Autodesk Inventor part; units mm, degrees
ref_plane "YZ Plane" through (0, 0, 0) normal (1, 0, 0) x (0, 1, 0)
ref_plane "XZ Plane" through (0, 0, 0) normal (0, 1, 0) x (-1, 0, 0)
ref_plane "XY Plane" through (0, 0, 0) normal (0, 0, 1) x (1, 0, 0)
sketch "Sketch1" plane through (0, 0, 0) normal (0, 1, 0) x (-1, 0, 0)
  circle A0 centre (0, 0) radius 25
  line L0 (10, 1.5) -> (-10, 1.5)
  line L1 (-10, 1.5) -> (-10, -1.5)
  line L2 (-10, -1.5) -> (10, -1.5)
  line L3 (10, -1.5) -> (10, 1.5)
  line L4 (1.5, 10) -> (-1.5, 10)
  line L5 (-1.5, 10) -> (-1.5, -10)
  line L6 (-1.5, -10) -> (1.5, -10)
  line L7 (1.5, -10) -> (1.5, 10)
  point P0 (-1.5, 1.5)
  point P1 (1.5, 1.5)
  point P2 (1.5, -1.5)
  point P3 (-1.5, -1.5)
  dimension "d0" = 50
  dimension "d1" = 20
  dimension "d2" = 3
  dimension "d3" = 1.5
  dimension "d4" = 10
  dimension "d5" = 3
  dimension "d6" = 20
  dimension "d7" = 10
  dimension "d8" = 1.5
extrude "Extrusion1" add sketch "Sketch1" along normal blind 3
properties part number "Base Arvore"
Verification items for the finished model (mm, model axes). A direction names the side the tool comes from. Give positions to 0.01 mm unless a question says otherwise; leave off trailing zeros. Write each loop counter-clockwise with the first axis right and the second up, starting at its lowest first coordinate (ties: lowest second). Pieces come first, ordered by that corner, then holes. Notation, with made-up numbers: (59.25, 7.25) - (82.25, 7.25) arc R10 ccw to (82.25, 22.25) - close; hole circle Ø9 at (10.5, 66.25). An arc over 180 degrees is marked (long way). Put each result on its own line as item: value.
Q1. Section check A-A on x = 0. Record the cut outline in (y, z).
Result:
outline: (0, -25) - (3, -25) - (3, -10) - (0, -10) - close; (0, 10) - (3, 10) - (3, 25) - (0, 25) - close
Q2. Set-up check for faces 1 (the face through (-5, 0, -5)), 2 (the face through (10, 1, 0)): record each of +Z, -Z, +X, -X, +Y, -Y from which the full face is reachable in a straight line by a thin tool's end or side.
Result:
face 1: +Z, -Z, +X, -X, -Y
face 2: +Y, -Y
Q3. Section check C-C on y = 2. Record the cut outline in (x, z).
Result:
outline: circle Ø50 at (0, 0); hole (-10, -1.5) - (-1.5, -1.5) - (-1.5, -10) - (1.5, -10) - (1.5, -1.5) - (10, -1.5) - (10, 1.5) - (1.5, 1.5) - (1.5, 10) - (-1.5, 10) - (-1.5, 1.5) - (-10, 1.5) - close
Q4. Mould release check, pull along X, two halves, no side actions. Record for faces 3 (the face through (-5, 3, -5)), 4 (the face through (-23.846, 1.479, -7.509)), 5 (the face through (6, 1, -1.5)): released by +X, released by -X, zero draft, split by the parting line, or undercut.
Result:
face 3: zero draft
face 4: split by the parting line
face 5: undercut
Q5. Depth check by flat-ended pin: P1, Ø1.5, axis at x = 0, y = 1, coming from the -Z side; P2, Ø0.9, axis at x = -0.5, y = 2, coming from the +Z side; P3, Ø0.9, axis at y = 2, z = -4.5, coming from the +X side. Enter the tip coordinate at first touch or a pass-through.
Result:
P1: z = -25
P2: z = 25
P3: x = 24.67
Q6. Section check B-B on z = 0. Record the cut outline in (x, y), and give its area (3 significant figures).
Result:
outline: (-25, 0) - (-10, 0) - (-10, 3) - (-25, 3) - close; (10, 0) - (25, 0) - (25, 3) - (10, 3) - close
area: 90.0 mm2
Q7. Scan lines: probe 1 along X at (y, z) = (2.9, 1); probe 2 along X at (y, z) = (0.45, -6); probe 3 along Z at (x, y) = (-2, 1.35). Record each from-to range of solid material in increasing order. Write a range as from..to.
Result:
probe 1: -24.98..-10, 10..24.98
probe 2: -24.27..-1.5, 1.5..24.27
probe 3: -24.92..-1.5, 1.5..24.92
Q8. Section check D-D on x = 16. Record the cut outline in (y, z), and give its area (3 significant figures).
Result:
outline: (0, -19.21) - (3, -19.21) - (3, 19.21) - (0, 19.21) - close
area: 115 mm2
